Geometry check sheet. Reference: drawing and pictorial views, mm from the part's lowest x, y, z. Give positions to 0.01 mm unless a question says otherwise; leave off trailing zeros. Order: outer loops, then holes, each group sorted by start corner. A loop starts at its lowest first (then second) coordinate and runs counter-clockwise, first axis right, second up. Notation, with made-up numbers: M 6,-2.5 L 49,-2.5 A25 cw 49,36.5 Z; hole C 15,25 d11. An arc over 180 degrees is marked long. Use CSV: the item, a comma, the result in double quotes. Start each with the question number.
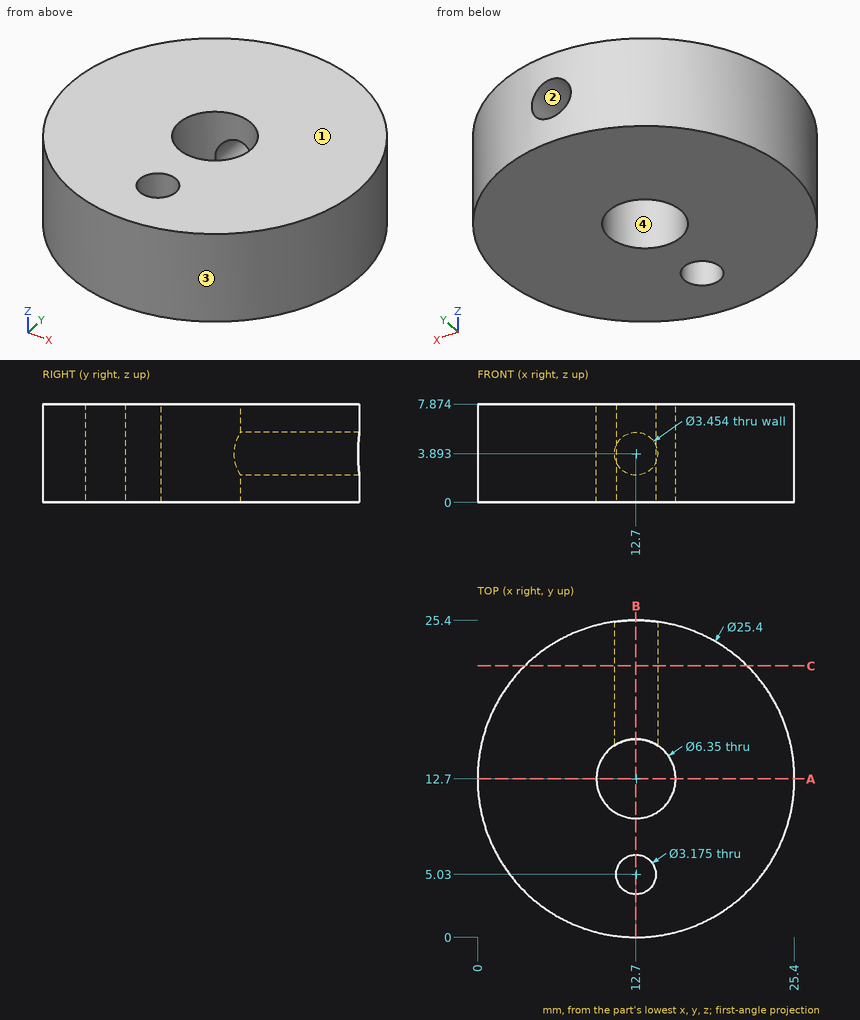
(1) Sectioned sample at A-A on y = 12.7. Record the cut outline in (x, z) (1 decimal), then the cut area to 3 significant figures.
(2) Draft check along X on the marked faces 1, 2, 3 and 4. Enter one of: +X half, -X half, draft (parallel to the pull), parting line (faces both ways), or undercut.
(3) Sectioned sample at B-B on x = 12.7. Record the cut outline in (y, z) (1 decimal).
(4) Go/stop test with flat-tipped pins: P1, Ø2, axis at x = 12.7, z = 3.89, coming from the +Y side; P2, Ø2, axis at y = 17.5, z = 5, coming from the -X side; P3, Ø1, axis at y = 13.5, z = 2, coming from the -X side. Record where each tip stops, or that it passes through.
(5) Thickness scan on line 1 (Y direction, x = 12.7, z = 6.25) (1 decimal); line 2 (X direction, y = 12.75, z = 3.75) (1 decimal); line 3 (Y direction, x = 12.7, z = 3.5) (1 decimal). Record the ranges inside material, lowest first.
(6) Sectioned sample at C-C on y = 21.75. Record the cut outline in (x, z) (1 decimal).
Responses:
1,outline,"M 0,0 L 9.5,0 L 9.5,7.9 L 0,7.9 Z; M 15.9,0 L 25.4,0 L 25.4,7.9 L 15.9,7.9 Z"
1,area,"150 mm2"
2,face 1,"draft"
2,face 2,"undercut"
2,face 3,"parting line"
2,face 4,"undercut"
3,outline,"M 0,0 L 3.4,0 L 3.4,7.9 L 0,7.9 Z; M 6.6,0 L 9.5,0 L 9.5,7.9 L 6.6,7.9 Z; M 15.9,0 L 25.4,0 L 25.4,2.2 L 15.9,2.2 Z; M 15.9,5.6 L 25.4,5.6 L 25.4,7.9 L 15.9,7.9 Z"
4,P1,"y = 9.69"
4,P2,"x = 0.58"
4,P3,"x = 0"
5,line 1,"0 to 3.4, 6.6 to 9.5, 15.9 to 25.4"
5,line 2,"0 to 9.5, 15.9 to 25.4"
5,line 3,"0 to 3.4, 6.6 to 9.5"
6,outline,"M 3.8,0 L 21.6,0 L 21.6,7.9 L 3.8,7.9 Z; hole C 12.7,3.9 d3.5"
